```python
from build123d import *

# Parameters (mm, degrees)
M3X0_5_TAPPED_HOLE1_D = 2.5
CUT_EXTRUDE1_REACH    = 8.563
CIRPATTERN1_COUNT     = 20


with BuildPart() as part:
    # Sketch1 → Revolve1 (revolve)
    with BuildSketch(Plane.XY, mode=Mode.PRIVATE) as revolve1_sk:
        Polygon((-2.85, 0), (2.85, 0), (2.85, 2.3), (1.35, 2.3), (1.35, 2), (0.45, 2), (0.45, 2.3), (-1.05, 2.3), (-1.05, 1.8), (-1.75, 1.8), (-1.75, 2), (-2.85, 2), align=None)
    revolve(revolve1_sk.sketch.rotate(Axis((-2.85, 0, 0), (1, 0, 0)), 180), axis=Axis((-2.85, 0, 0), (1, 0, 0)))

    # M3x0.5 Tapped Hole1 (through all)
    with Locations(Plane(origin=(2.85, 0, 0), x_dir=(0, 0, -1), z_dir=(1, 0, 0))):
        with Locations((0, 0)):
            Hole(M3X0_5_TAPPED_HOLE1_D / 2)

    # Cut-Extrude1: up to this face of the body (flat: up to its plane)
    cut_extrude1_end = Plane(part.part.faces().sort_by_distance((-1.05, 2.234946176, 0))[0])
    # Sketch4 → Cut-Extrude1 (cut, up to the picked face)
    with BuildSketch(Plane(origin=(2.85, 0, 0), x_dir=(0, 0, -1), z_dir=(1, 0, 0)), mode=Mode.PRIVATE) as cut_extrude1_sk1:
        with BuildLine():
            Line((0.229949273, 2.288476203), (0.15, 2.15))
            Line((0.15, 2.15), (-0.15, 2.15))
            Line((-0.15, 2.15), (-0.229949273, 2.288476203))
            ThreePointArc((-0.229949273, 2.288476203), (0, 2.3), (0.229949273, 2.288476203))
        make_face()
    cut_extrude1_tool1 = split(extrude(cut_extrude1_sk1.sketch, amount=-CUT_EXTRUDE1_REACH, mode=Mode.PRIVATE), bisect_by=cut_extrude1_end, keep=Keep.BOTH, mode=Mode.PRIVATE)
    cut_extrude1 = cut_extrude1_tool1.solids().sort_by(Axis((2.85, 2.228438, 0), (-1, 0, 0)))[0]
    add(cut_extrude1, mode=Mode.SUBTRACT)

    # CirPattern1: Cut-Extrude1 ×20 about axis
    cirpattern1_axis = Axis((0, 0, 0), (1, 0, 0))
    for i in range(1, CIRPATTERN1_COUNT):
        add(cut_extrude1.rotate(cirpattern1_axis, i * 360 / CIRPATTERN1_COUNT), mode=Mode.SUBTRACT)


solid = part.part
```
Could you check a few things on this model? Use its own coordinates, in mm. A direction names the side the tool comes from. Give positions to 0.01 mm unless a question says otherwise; leave off trailing zeros. Loops run counter-clockwise (first coordinate to the right, second up) from the corner with the lowest first, then second, coordinate; pieces in that order, holes last. Notation, with made-up numbers: (17.25, 32.25) -> (26.25, 32.25) arc R20 ccw to (26.25, 47.25) -> close; hole circle Ø10 at (8.25, 32). An arc over 180 degrees is marked (long way). Put each result on its own line as item: value.
(1) Thinking about a two-plate mould opening in Y: for faces 1 (the face through (2.85, 1, 1)), 2 (the face through (-1.405, -1.717, -0.541)), 3 (the face through (-0.04, -1.22, -0.27)), which applies, pulls with the +Y half, pulls with the -Y half, needs draft (parallel to the pull), parting line crosses it, or undercut?
Computed:
face 1: needs draft
face 2: parting line crosses it
face 3: undercut
(2) Imagine slicing it at A-A on z = 0. Write out the boundary of the cut face in (x, y), plus the area to 3 significant figures.
Computed:
outline: (-2.85, -2) -> (-1.75, -2) -> (-1.75, -1.8) -> (-1.05, -1.8) -> (-1.05, -2.15) -> (0.45, -2.15) -> (0.45, -2) -> (1.35, -2) -> (1.35, -2.15) -> (2.85, -2.15) -> (2.85, -1.25) -> (-2.85, -1.25) -> close; (-2.85, 1.25) -> (2.85, 1.25) -> (2.85, 2.15) -> (1.35, 2.15) -> (1.35, 2) -> (0.45, 2) -> (0.45, 2.15) -> (-1.05, 2.15) -> (-1.05, 1.8) -> (-1.75, 1.8) -> (-1.75, 2) -> (-2.85, 2) -> close
area: 9.17 mm^2
(3) Imagine slicing it at C-C on x = -2.25. Write out the boundary of the cut face in (y, z), plus the area to 3 significant figures.
Computed:
outline: circle Ø4 at (0, 0); hole circle Ø2.5 at (0, 0)
area: 7.66 mm^2
(4) Please list where these lines run through material, in increasing order: probe 1 along Y at (x, z) = (-0.75, 0); probe 2 along X at (y, z) = (1.9, -1.05); probe 3 along X at (y, z) = (-1.9, -0.4). Write a range as [from, to].
Computed:
probe 1: [-2.15, -1.25], [1.25, 2.15]
probe 2: [-1.05, 0.45], [1.35, 2.85]
probe 3: [-2.85, -1.75], [-1.05, 2.85]
(5) For faces 4 (the face through (-2, 0, 2)), 5 (the face through (1, 0, 2)), 6 (the face through (-2.85, -1, -1)), which set-ups out of +Z, -Z, +X, -X, +Y, -Y let a thin tool reach every point of the face, with its end or its side?
Computed:
face 4: -X
face 5: none
face 6: +Z, -Z, -X, +Y, -Y
(6) Imagine slicing it at D-D on z = 1.9. Write out the boundary of the cut face in (x, y).
Computed:
outline: (-2.85, -0.62) -> (-1.75, -0.62) -> (-1.75, 0.62) -> (-2.85, 0.62) -> close; (-1.05, -1.15) -> (0.45, -1.15) -> (0.45, -0.62) -> (1.35, -0.62) -> (1.35, -1.15) -> (2.85, -1.15) -> (2.85, 1.15) -> (1.35, 1.15) -> (1.35, 0.62) -> (0.45, 0.62) -> (0.45, 1.15) -> (-1.05, 1.15) -> close
(7) I'm going to push flat-ended pins straight in: pin 1 Ø2 at (y, z) = (-1, 0) entering from +X; pin 2 Ø2 at (y, z) = (0, 0) entering from -X. Where does each tip first touch, or does it pass through?
Computed:
pin 1: x = 2.85
pin 2: through
